```python
from build123d import *

# Parameters (mm, degrees)
SKETCH1_R               = 62
BOSS_EXTRUDE1_DEPTH     = 5
SKETCH2_R               = 2
CUT_EXTRUDE1_DEPTH      = 5
CIRPATTERN1_COUNT       = 2
CIRPATTERN1_ANGLE       = 120
MIRROR1_COPY_1_SKETCH_R = 2
MIRROR1_COPY_1_DEPTH    = 5
SKETCH5_R               = 62
SKETCH5_R_2             = 57
BOSS_EXTRUDE2_DEPTH     = 8
CUT_EXTRUDE2_START      = -90
SKETCH6_R               = 1.5
CUT_EXTRUDE2_DEPTH      = 91
CIRPATTERN2_COUNT       = 5
SKETCH7_R               = 3
CUT_EXTRUDE3_DEPTH      = 10


with BuildPart() as part:
    # Sketch1 → Boss-Extrude1 (new body)
    with BuildSketch(Plane(origin=(0, 0, 0), x_dir=(1, 0, 0), z_dir=(0, 1, 0))):
        with Locations(Location((0, 0, 0), (0, 0, 270))):
            Circle(SKETCH1_R)
    extrude(amount=BOSS_EXTRUDE1_DEPTH)

    # Sketch2 → Cut-Extrude1 (cut)
    with BuildSketch(Plane(origin=(0, 5, 0), x_dir=(1, 0, 0), z_dir=(0, 1, 0))):
        with Locations(Location((0, 49.5, 0), (0, 0, 270))):
            Circle(SKETCH2_R)
    cut_extrude1 = extrude(amount=-CUT_EXTRUDE1_DEPTH, mode=Mode.SUBTRACT)

    # CirPattern1: Cut-Extrude1 ×2 about axis
    cirpattern1_axis = Axis((0, 5, 0), (0, 1, 0))
    for i in range(1, CIRPATTERN1_COUNT):
        add(cut_extrude1.rotate(cirpattern1_axis, i * CIRPATTERN1_ANGLE / (CIRPATTERN1_COUNT - 1)), mode=Mode.SUBTRACT)

    # Mirror1: Cut-Extrude1 across plane
    add(cut_extrude1.mirror(Plane(origin=(0, 0, 0), x_dir=(-0.49999999999999806, 0, 0.8660254037844398), z_dir=(-0.8660254037844398, 0, -0.49999999999999806))), mode=Mode.SUBTRACT)

    # Mirror1 copy 1 sketch → Mirror1 copy 1 (cut)
    with BuildSketch(Plane(origin=(0, 5, 0), x_dir=(1, 0, 0), z_dir=(0, 1, 0))):
        with Locations((0, -49.5)):
            Circle(MIRROR1_COPY_1_SKETCH_R)
    extrude(amount=-MIRROR1_COPY_1_DEPTH, mode=Mode.SUBTRACT)

    # Sketch5 → Boss-Extrude2 (add)
    with BuildSketch(Plane(origin=(0, 5, 0), x_dir=(1, 0, 0), z_dir=(0, 1, 0))):
        with Locations(Location((0, 0, 0), (0, 0, 270))):
            Circle(SKETCH5_R)
        with Locations(Location((0, 0, 0), (0, 0, 270))):
            Circle(SKETCH5_R_2, mode=Mode.SUBTRACT)
    extrude(amount=BOSS_EXTRUDE2_DEPTH)

    # Sketch6 → Cut-Extrude2 (cut)
    with BuildSketch(Plane(origin=(0, 0, 0), x_dir=(-0.49999999999999806, 0, 0.8660254037844398), z_dir=(-0.8660254037844398, 0, -0.49999999999999806)).offset(CUT_EXTRUDE2_START)):
        with Locations(Location((0, 7, 0), (0, 0, 180))):
            Circle(SKETCH6_R)
    cut_extrude2 = extrude(amount=CUT_EXTRUDE2_DEPTH, mode=Mode.SUBTRACT)

    # CirPattern2: Cut-Extrude2 ×5 about axis
    cirpattern2_axis = Axis((0, 13, 0), (0, 1, 0))
    for i in range(1, CIRPATTERN2_COUNT):
        add(cut_extrude2.rotate(cirpattern2_axis, i * 360 / CIRPATTERN2_COUNT), mode=Mode.SUBTRACT)

    # Sketch7 → Cut-Extrude3 (cut)
    with BuildSketch(Plane(origin=(0, 5, 0), x_dir=(1, 0, 0), z_dir=(0, 1, 0))):
        with Locations(Location((0, 0, 0), (0, 0, 270))):
            Circle(SKETCH7_R)
    extrude(amount=-CUT_EXTRUDE3_DEPTH, mode=Mode.SUBTRACT)


solid = part.part
```
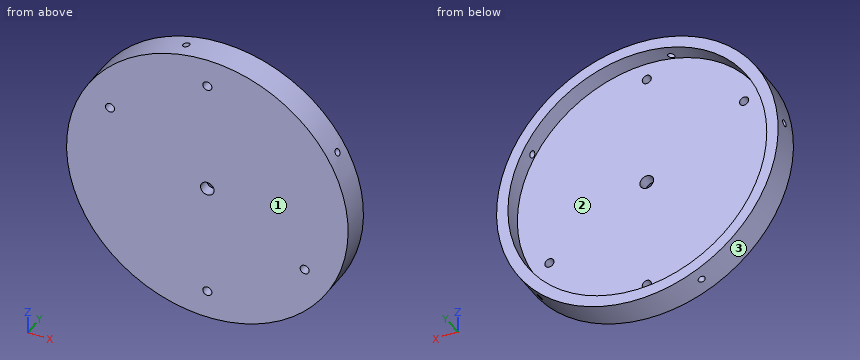
Here's how the part is built. I have some questions about the finished solid (model axes, mm). Face numbers are marked on the shaded views. Coordinates: 2 decimals unless noted, no trailing zeros. Order: outer loops, then holes, each group sorted by start corner. A loop starts at its lowest first (then second) coordinate and runs counter-clockwise, first axis right, second up. Notation, with made-up numbers: M -17,66 L 9,66 A19 ccw 9,88 Z; hole C 21.25,-27 d9. An arc over 180 degrees is marked long. Answer as a JSON object with one key per item and string values. Group by question number.
(1) Suppose I cut it at A-A, the plane z = 0. Please give me the cut outline in (x, y).
(2) I need wall thicknesses on probe 1 along Y at (x, z) = (14.5, 40); probe 2 along X at (y, z) = (7.25, 0); probe 3 along X at (y, z) = (6.5, 44). Which ranges of each line are inside material? Lowest first, please.
(3) Suppose I cut it at C-C, the plane z = -49.5. Please give me the cut outline in (x, y).
(4) For pin 1 (2.5 mm diameter, centred on x = 0, z = 49.5, fed in from -Y); pin 2 (6.5 mm diameter, centred on x = 42.87, z = -24.75, fed in from +Y); pin 3 (1.5 mm diameter, centred on x = 40, y = 2, fed in from +Z); pin 4 (4 mm diameter, centred on y = 5, z = 2, fed in from -X), each with a flat end and sliding along its axis, tell me the tip position at first contact or that it passes through.
(5) Suppose I cut it at B-B, the plane x = -53.5. Please give me the cut outline in (y, z), then the cut area to 3 significant figures.
(6) If we mould it in two halves opening along Z, with no side actions, what happens to the marked faces 1, 2 and 3? For each: released by +Z, released by -Z, zero draft, split by the parting line, or undercut.
(7) Suppose I cut it at D-D, the plane x = -17. Please give me the cut outline in (y, z).
Values found:
{
 "1": {"outline": "M -62,0 L -3,0 L -3,5 L -57,5 L -57,13 L -62,13 Z; M 3,0 L 62,0 L 62,13 L 57,13 L 57,5 L 3,5 Z"},
 "2": {"probe 1": "y = 0 to 5", "probe 2": "x = -62 to -57, 57 to 62", "probe 3": "x = -43.68 to -36.24, 36.24 to 43.68"},
 "3": {"outline": "M -37.33,0 L -2,0 L -2,5 L -28.26,5 L -28.26,13 L -37.33,13 Z; M 2,0 L 37.33,0 L 37.33,13 L 28.26,13 L 28.26,5 L 2,5 Z"},
 "4": {"pin 1": "passes through", "pin 2": "stops at y = 5", "pin 3": "stops at z = 47.99", "pin 4": "stops at x = -62"},
 "5": {"outline": "M 0,-31.33 L 13,-31.33 L 13,-19.67 L 5,-19.67 L 5,19.67 L 13,19.67 L 13,31.33 L 0,31.33 Z", "area": "500 mm^2"},
 "6": {"face 1": "zero draft", "face 2": "undercut", "face 3": "split by the parting line"},
 "7": {"outline": "M 0,-59.62 L 13,-59.62 L 13,-54.41 L 5,-54.41 L 5,54.41 L 13,54.41 L 13,59.62 L 0,59.62 Z"}
}
